CAD build for the part. Positions are in the model's coordinates, mm. Face numbers are marked on the shaded views. A direction names the side the tool comes from. Round coordinates to 2 decimals unless told otherwise and drop trailing zeros. Loops run counter-clockwise (first coordinate to the right, second up) from the corner with the lowest first, then second, coordinate; pieces in that order, holes last. Notation, with made-up numbers: M 80,-20 L 94,-20 A11 cw 94,-15 Z; hole C 46.5,11.25 d3. An arc over 180 degrees is marked long. Put each result on its own line as item: value. Start each with the question number.
from build123d import *

# Parameters (mm, degrees)
SKETCH1_W           = 26
SKETCH1_H           = 26
BOSS_EXTRUDE1_DEPTH = 15
CHAMFER1_SIZE       = 5
CHAMFER1_SIZE2      = 8.660254038
SKETCH2_W           = 8
SKETCH2_H           = 2
BOSS_EXTRUDE2_DEPTH = 8
FILLET1_R           = 4
CUT_EXTRUDE2_REACH  = 80.899
SKETCH5_R           = 1.55


with BuildPart() as part:
    # Sketch1 → Boss-Extrude1 (new body)
    with BuildSketch(Plane.XY):
        with Locations((57, 13)):
            Rectangle(SKETCH1_W, SKETCH1_H)
    extrude(amount=BOSS_EXTRUDE1_DEPTH)

    # Chamfer1
    chamfer1_edges = [part.edges().sort_by_distance(p)[0] for p in [
        (57, 26, 15),
    ]]
    chamfer1_side = [part.faces().sort_by_distance(p)[0] for p in [
        (57, 26, 7.5),
    ]]
    chamfer(chamfer1_edges, length=CHAMFER1_SIZE, length2=CHAMFER1_SIZE2, reference=chamfer1_side[0])

    # Sketch2 → Boss-Extrude2 (add)
    with BuildSketch(Plane(origin=(0, 26, 0), x_dir=(1, 0, 0), z_dir=(0, 1, 0))):
        with Locations((48, -1)):
            Rectangle(SKETCH2_W, SKETCH2_H)
        with Locations((66, -1)):
            Rectangle(SKETCH2_W, SKETCH2_H)
    extrude(amount=BOSS_EXTRUDE2_DEPTH)

    # Fillet1
    fillet1_edges = [part.edges().sort_by_distance(p)[0] for p in [
        (44, 34, 1),
        (52, 34, 1),
        (62, 34, 1),
        (70, 34, 1),
    ]]
    fillet(fillet1_edges, radius=FILLET1_R - 0.0001)  # a hair under: the kernel refuses the full size

    # Sketch5 → Cut-Extrude2 (cut, up to next)
    with BuildSketch(Plane.XY.offset(2), mode=Mode.PRIVATE) as cut_extrude2_sk1:
        with Locations((66, 30)):
            Circle(SKETCH5_R)
    cut_extrude2_tool1 = extrude(cut_extrude2_sk1.sketch, amount=-CUT_EXTRUDE2_REACH, mode=Mode.PRIVATE) & part.part
    # Sketch5 → Cut-Extrude2 (cut, up to next)
    with BuildSketch(Plane.XY.offset(2), mode=Mode.PRIVATE) as cut_extrude2_sk2:
        with Locations((48, 30)):
            Circle(SKETCH5_R)
    cut_extrude2_tool2 = extrude(cut_extrude2_sk2.sketch, amount=-CUT_EXTRUDE2_REACH, mode=Mode.PRIVATE) & part.part
    add(cut_extrude2_tool1.solids().sort_by_distance((66, 30, 2))[0], mode=Mode.SUBTRACT)
    add(cut_extrude2_tool2.solids().sort_by_distance((48, 30, 2))[0], mode=Mode.SUBTRACT)


solid = part.part
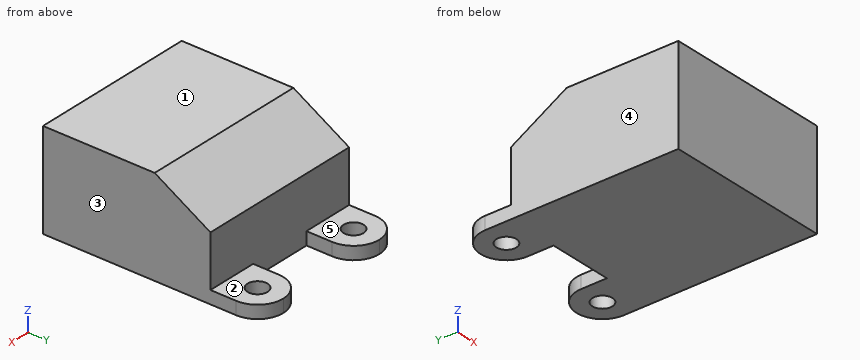
(1) Drill centre lines: line 1 along Y through (x, z) = (48, 1.5); line 2 along Y through (x, z) = (59, 1.5); line 3 along Z through (x, y) = (61.5, 25). Where is each one in solid material? Low to high.
(2) Cut at C-C on x = 51. List the corners of the cut face in (y, z), and give its area (3 significant figures).
(3) Mould opens along X. For the marked faces 3, 4 and 5 say: +X half, -X half, draft (parallel to the pull), parting line (faces both ways), or undercut.
(4) Cut at A-A on y = 26.5. List the corners of the cut face in (x, z), and give its area (3 significant figures).
(5) Tool access for the marked faces 1 and 2: list every direction of +Z, -Z, +X, -X, +Y, -Y with a clear straight run to the whole face (end or side of a thin tool).
(6) Flat gauge pins, fed straight in: pin 1 Ø4 at (x, y) = (48, 29.5) entering from +Z; pin 2 Ø1 at (x, z) = (48, 5) entering from +Y; pin 3 Ø3 at (x, y) = (66, 30) entering from -Z. Where does each tip first touch, or does it go through?
(7) Cut at B-B on y = 31. List the corners of the cut face in (x, z), and give its area (3 significant figures).
(8) Cut at D-D on z = 8.5. List the corners of the cut face in (x, y).
Taken from the geometry:
1. line 1: 0 to 28.45, 31.55 to 34
1. line 2: 0 to 26
1. line 3: 0 to 10.58
2. outline: M 0,0 L 32.65,0 L 32.65,2 L 26,2 L 26,10 L 17.34,15 L 0,15 Z
2. area: 382 mm2
3. face 3: +X half
3. face 4: -X half
3. face 5: draft
4. outline: M 44,0 L 52,0 L 52,2 L 44,2 Z; M 62,0 L 70,0 L 70,2 L 62,2 Z
4. area: 32.0 mm2
5. face 1: +Z, +X, -X, +Y, -Y
5. face 2: +Z, +X, -X, +Y
6. pin 1: z = 2
6. pin 2: y = 26
6. pin 3: through
7. outline: M 44.13,0 L 46.82,0 L 46.82,2 L 44.13,2 Z; M 49.18,0 L 51.87,0 L 51.87,2 L 49.18,2 Z; M 62.13,0 L 64.82,0 L 64.82,2 L 62.13,2 Z; M 67.18,0 L 69.87,0 L 69.87,2 L 67.18,2 Z
7. area: 21.5 mm2
8. outline: M 44,0 L 70,0 L 70,26 L 44,26 Z
